```python
from build123d import *

# Parameters (mm, degrees)
F0_R      = 32.5
F1_DEPTH  = 2
F3_DEPTH  = 16
F5_DEPTH  = 5
F8_DEPTH  = 3.5
F10_DEPTH = 6.5
F12_DEPTH = 5


with BuildPart() as f1:
    # F0 (on Top) → F1 (new body)
    with BuildSketch(Plane.XY):
        Circle(F0_R)
    extrude(amount=F1_DEPTH)

    # F2 (on face) → F3 (join)
    with BuildSketch(Plane.XY.offset(2)):
        Polygon((-17.470987, 26.293807), (-29.398278, 11.503954), (-24.727798, 7.737442), (-19.078029, 14.743161), (-19.856442, 15.370914), (-19.22869, 16.149327), (-18.450276, 15.521575), (-12.800507, 22.527294), align=None)
        Polygon((9.5, 30.105642), (-9.5, 30.105642), (-9.5, 24.105642), (-0.5, 24.105642), (-0.5, 25.105642), (0.5, 25.105642), (0.5, 24.105642), (9.5, 24.105642), align=None)
        Polygon((-31.434899, 2.906345), (-27.409662, -15.662378), (-21.545855, -14.391251), (-23.452546, -5.59554), (-24.429847, -5.807395), (-24.641702, -4.830094), (-23.664401, -4.618239), (-25.571091, 4.177472), align=None)
        Polygon((26.734962, -6.679754), (19.490518, -4.738611), (17.549375, -11.983055), (24.793819, -13.924198), align=None)
    extrude(amount=F3_DEPTH)

    # F4 (on face) → F5 (join)
    with BuildSketch(Plane.XY.offset(2)):
        Polygon((10.338692, -4.986162), (-7.925741, -5.943361), (-7.623178, -11.7166), (10.641255, -10.759402), align=None)
        Polygon((9.017375, 16.199804), (-9.247058, 15.242605), (-8.944496, 9.469366), (9.319937, 10.426564), align=None)
    extrude(amount=F5_DEPTH)

    # F7 (on face) → F8 (join)
    with BuildSketch(Plane.XY.offset(2)):
        Polygon((3.241127, 7.73687), (-2.750651, 7.422854), (-2.436635, 1.431077), (3.555142, 1.745093), align=None)
        Polygon((4.577761, -14.010625), (-1.414016, -14.324641), (-1.1, -20.316418), (4.891777, -20.002403), align=None)
    extrude(amount=F8_DEPTH)

    # F9 (on face) → F10 (join)
    with BuildSketch(Plane.XY.offset(5.5)):
        Polygon((3.45047, 3.742352), (-2.541307, 3.428336), (-2.436635, 1.431077), (3.555142, 1.745093), align=None)
        Polygon((4.787105, -18.005143), (-1.204672, -18.319159), (-1.1, -20.316418), (4.891777, -20.002403), align=None)
    extrude(amount=F10_DEPTH)

    # F11 (on face) → F12 (join)
    with BuildSketch(Plane.XY.offset(7)):
        Polygon((-3.905181, -6.876087), (-7.291749, -9.004739), (-6.493505, -10.274702), (-3.106937, -8.14605), align=None)
        Polygon((4.006315, -6.182721), (-1.985463, -6.496736), (-1.906959, -7.994681), (4.084819, -7.680665), align=None)
        Polygon((9.730671, -7.986948), (5.980971, -6.594201), (5.458691, -8.000339), (9.208391, -9.393086), align=None)
        Polygon((-4.832129, 14.484637), (-8.218697, 12.355986), (-7.420453, 11.086022), (-4.033884, 13.214674), align=None)
        Polygon((2.746676, 15.221225), (-3.245101, 14.907209), (-3.166597, 13.409265), (2.82518, 13.72328), align=None)
        Polygon((7.883003, 13.715759), (4.133302, 15.108505), (3.611022, 13.702367), (7.360723, 12.309621), align=None)
    extrude(amount=F12_DEPTH)


solid = f1.part
```
Can you work these out from the model? Positions are in its coordinate system, mm. A direction names the side the tool comes from. Coordinates: 2 decimals unless noted, no trailing zeros. Order: outer loops, then holes, each group sorted by start corner. A loop starts at its lowest first (then second) coordinate and runs counter-clockwise, first axis right, second up.
1. I need wall thicknesses on line 1 (Y direction, x = 7.5, z = 3.25); line 2 (Z direction, x = -20.5, y = -5); line 3 (Y direction, x = -26, z = 5.5). Which ranges of each line are inside material? Lowest first, please.
2. Thinking about a two-plate mould opening in Y: for faces 6 (the face through (18.534, -8.31, 9.888)), 7 (the face through (0.517, 1.586, 6.93)), 8 (the face through (9.466, -8.7, 9.465)), which applies, +Y half, -Y half, draft (parallel to the pull), parting line (faces both ways), or undercut?
3. If we section it at A-A (z = 15): Please give me the cut outline in (x, y).
4. For faces 1 (the face through (1, -7, 12)), 2 (the face through (-24.6, -0.3, 9.9)), 3 (the face through (3.4, 4.7, 3.7)), 4 (the face through (-9.5, 27, 10)), 5 (the face through (1.85, -20.16, 6.93)), which set-ups out of +Z, -Z, +X, -X, +Y, -Y let a thin tool reach every point of the face, with its end or its side?
5. If we section it at D-D (z = 2.75): Give the number of separate pieces and of enclosed holes in the cut face, then the cut area to 3 significant figures.
6. If we section it at B-B (x = -26.5): Please give me the cut outline in (y, z).
7. I'm going to push flat-ended pins straight in: pin 1 (7 mm diameter, centred on x = -4.5, z = 10.5, fed in from -Y); pin 2 (0.9 mm diameter, centred on x = -1.5, y = 14.5, fed in from +Z); pin 3 (4.5 mm diameter, centred on x = 2, y = -15.5, fed in from +Z). Where does each tip first touch, or does it pass through?
8. If we section it at C-C (y = 18.5): Please give me the cut outline in (x, z), then the cut area to 3 significant figures.
Entries:
1. line 1: y = -10.92 to -5.13, 10.33 to 16.12, 24.11 to 30.11
1. line 2: z = 0 to 2
1. line 3: y = -15.36 to 4.08, 8.76 to 15.72
2. face 6: +Y half
2. face 7: undercut
2. face 8: -Y half
3. outline: (-31.43, 2.91) - (-27.41, -15.66) - (-21.55, -14.39) - (-23.45, -5.6) - (-24.43, -5.81) - (-24.64, -4.83) - (-23.66, -4.62) - (-25.57, 4.18) - close; (-29.4, 11.5) - (-24.73, 7.74) - (-19.08, 14.74) - (-19.86, 15.37) - (-19.23, 16.15) - (-18.45, 15.52) - (-12.8, 22.53) - (-17.47, 26.29) - close; (-9.5, 24.11) - (-0.5, 24.11) - (-0.5, 25.11) - (0.5, 25.11) - (0.5, 24.11) - (9.5, 24.11) - (9.5, 30.11) - (-9.5, 30.11) - close; (17.55, -11.98) - (24.79, -13.92) - (26.73, -6.68) - (19.49, -4.74) - close
4. face 1: +Z, -Y
4. face 2: +Z
4. face 3: +Z, +X
4. face 4: +Z, +Y, -Y
4. face 5: +Z, +X, -Y
5. separate pieces: 8
5. enclosed holes: 0
5. area: 679 mm2
6. outline: (-18.81, 0) - (18.81, 0) - (18.81, 2) - (15.1, 2) - (15.1, 18) - (9.17, 18) - (9.17, 2) - (3.98, 2) - (3.98, 18) - (-15.47, 18) - (-15.47, 2) - (-18.81, 2) - close
7. pin 1: stops at y = -20.32
7. pin 2: stops at z = 12
7. pin 3: stops at z = 5.5
8. outline: (-26.72, 0) - (26.72, 0) - (26.72, 2) - (-16.05, 2) - (-16.05, 18) - (-23.76, 18) - (-23.76, 2) - (-26.72, 2) - close
8. area: 230 mm2
